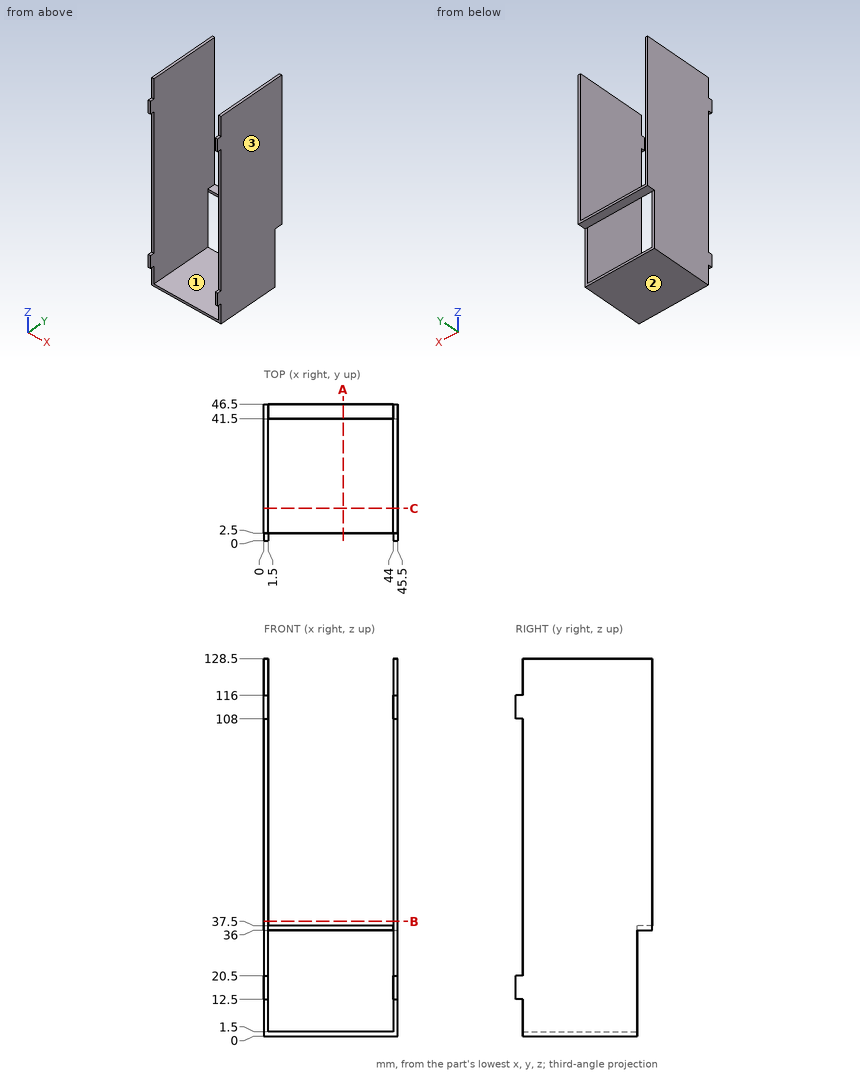
Can you work these out from the drawing? Everything is in mm from the part's minimum corner. Round coordinates to 2 decimals unless told otherwise and drop trailing zeros. Loops run counter-clockwise (first coordinate to the right, second up) from the corner with the lowest first, then second, coordinate; pieces in that order, holes last. Notation, with made-up numbers: M 9,-17.5 L 18,-17.5 A14 cw 18,5.5 Z; hole C -21.75,58.25 d4. An arc over 180 degrees is marked long. Write item = value, one per line.
1. I want a section at C-C, the plane y = 11. Write out the boundary of the cut face in (x, z), and give its area (3 significant figures).
Results below:
outline = M 0,0 L 45.5,0 L 45.5,128.5 L 44,128.5 L 44,1.5 L 1.5,1.5 L 1.5,128.5 L 0,128.5 Z
area = 449 mm²
2. I want a section at B-B, the plane z = 39. Write out the boundary of the cut face in (x, y), and give its area (3 significant figures).
Results below:
outline = M 0,2.5 L 1.5,2.5 L 1.5,46.5 L 0,46.5 Z; M 44,2.5 L 45.5,2.5 L 45.5,46.5 L 44,46.5 Z
area = 132 mm²
3. I need wall thicknesses on probe 1 along X at (y, z) = (17, 24); probe 2 along Z at (x, y) = (21, 31). Which ranges of each line are inside material? Lowest first, please.
Results below:
probe_1 = 0 to 1.5, 44 to 45.5
probe_2 = 0 to 1.5
4. I want a section at A-A, the plane x = 27. Write out the boundary of the cut face in (y, z), and give its area (3 significant figures).
Results below:
outline = M 2.5,0 L 41.5,0 L 41.5,1.5 L 2.5,1.5 Z; M 41.5,36 L 46.5,36 L 46.5,37.5 L 41.5,37.5 Z
area = 66.0 mm²
5. Thinking about a two-plate mould opening in X: for the marked faces 1, 2 and 3, which applies, +X half, -X half, draft (parallel to the pull), parting line (faces both ways), or undercut?
Results below:
face_1 = undercut
face_2 = draft
face_3 = +X half
6. Will these pins go through, and if not, where does the flat tip stop? P1, Ø1.6, axis at x = 22, z = 37, coming from the -Y side; P2, Ø0.8, axis at x = 45, y = 1.5, coming from the +Z side; P3, Ø5.5, axis at x = 13.5, y = 43, coming from the +Z side.
Results below:
P1 = 41.5
P2 = 116
P3 = 37.5
